Read the model definition and answer for the solid it produces. Units are mm, in the model's axes. Give positions to 0.01 mm unless a question says otherwise; leave off trailing zeros. Loops run counter-clockwise (first coordinate to the right, second up) from the corner with the lowest first, then second, coordinate; pieces in that order, holes last. Notation, with made-up numbers: (-15, -37) - (36, -37) arc R18 cw to (36, -16) - close; hole circle Ø2 at (79, 40.25). An arc over 180 degrees is marked (long way). Put each result on its own line as item: value. Start each with the question number.
1. Consider L1, parallel to X at y = 4.5, z = 18; L2, parallel to Y at x = 0, z = 18.75; L3, parallel to X at y = 3.5, z = 12. Determine where each line is inside the solid, lowest interval first. Write a range as from..to.
2. A cutting plane is placed at A-A, the plane y = 4.5. Determine the outline of the cut face in (x, z), plus the area to 3 significant figures.
3. A cutting plane is placed at B-B, the plane x = 0. Determine the outline of the cut face in (y, z).
Solid Edge part; units mm, degrees
sketch "Sketch1" plane through (0, 0, 0) normal (0, 0, 1) x (1, 0, 0)
  line L0 (-3, -7.5) -> (3, -7.5)
  line L1 (3, -7.5) -> (3, 7.5)
  line L2 (3, 7.5) -> (-3, 7.5)
  line L3 (-3, 7.5) -> (-3, -7.5)
  dimension "D1" = 3
  dimension "D2" = 3
extrude "Ajout_matière_1" add sketch "Sketch1" along normal blind 22
hole "Perçage_1" [suppressed]
hole "Perçage_2" [suppressed]
hole "Perçage_3" at (0, 4.5, 22) direction (0, 0, -1) diameter 2.459 depth 12 thread major 3 thread length 0.01
properties material "Plastique ABS, haute performance"
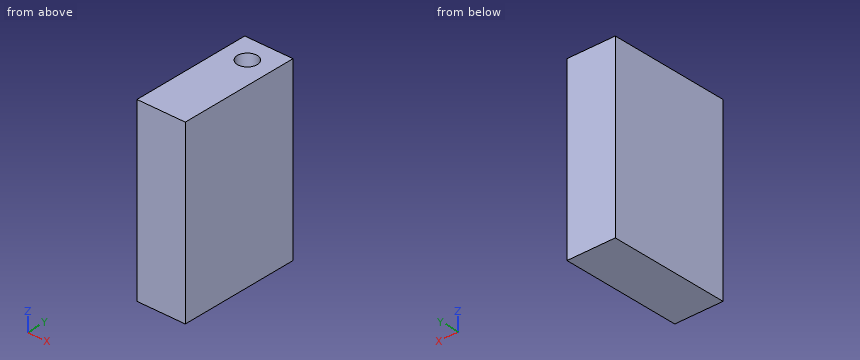
Return value:
1. L1: x = -3..-1.23, 1.23..3
1. L2: y = -7.5..3.27, 5.73..7.5
1. L3: x = -3..-0.72, 0.72..3
2. outline: (-3, 0) - (3, 0) - (3, 22) - (1.23, 22) - (1.23, 10) - (-1.23, 10) - (-1.23, 22) - (-3, 22) - close
2. area: 102 mm2
3. outline: (-7.5, 0) - (7.5, 0) - (7.5, 22) - (5.73, 22) - (5.73, 10) - (3.27, 10) - (3.27, 22) - (-7.5, 22) - close
